Design review of the part built by this model. Coordinates are the model's own, in mm. A direction names the side the tool comes from. Coordinates: 2 decimals unless noted, no trailing zeros. Order: outer loops, then holes, each group sorted by start corner. A loop starts at its lowest first (then second) coordinate and runs counter-clockwise, first axis right, second up. Notation, with made-up numbers: (37, 38.5) -> (90, 38.5) arc R23 cw to (90, 69.5) -> close; hole circle Ø5 at (27.5, -24.75). An arc over 180 degrees is marked (long way). Write item = value, one per line.
Autodesk Inventor part; units mm, degrees
ref_plane "YZ Plane" through (0, 0, 0) normal (1, 0, 0) x (0, 1, 0)
ref_plane "XZ Plane" through (0, 0, 0) normal (0, 1, 0) x (-1, 0, 0)
ref_plane "XY Plane" through (0, 0, 0) normal (0, 0, 1) x (1, 0, 0)
sketch "Sketch1" plane through (0, 0, 0) normal (1, 0, 0) x (0, 1, 0)
  line L0 (38, 32.5) -> (0, 32.5)
  line L1 (0, 32.5) -> (0, -32.5)
  line L2 (0, -32.5) -> (38, -32.5)
  line L3 (0, 0) -> (16.8405, 0)
  line L4 (38, 32.5) -> (38, 27.5)
  line L5 (29, 27.5) -> (5, 27.5)
  line L6 (5, 27.5) -> (5, -27.5)
  line L7 (5, -27.5) -> (29, -27.5)
  line L8 (5.264, 15) -> (-3.604, 15) construction
  line L9 (5.264, -15) -> (-3.604, -15) construction
  line L10 (38, 27.5) -> (36.5301, 27.5)
  line L11 (29, 30) -> (29, 27.5)
  line L12 (36.5301, 27.5) -> (32.2, 30)
  line L13 (32.2, 30) -> (29, 30)
  line L14 (38, -32.5) -> (38, -27.5)
  line L15 (38, -27.5) -> (36.5301, -27.5)
  line L16 (29, -30) -> (29, -27.5)
  line L17 (36.5301, -27.5) -> (32.2, -30)
  line L18 (32.2, -30) -> (29, -30)
  dimension "d0" = 5
  dimension "d1" = 30
  dimension "d2" = 65
  dimension "d3" = 38
  dimension "d5" = 3.2
  dimension "d6" = 24
  dimension "d7" = 2.5
  dimension "d8" = 30
  dimension "d9" = 5
  dimension "d10" = 5
  dimension "d30" = 60
extrude "Extrusion1" add sketch "Sketch1" along normal mid plane 15.1
sketch "Sketch2" plane through (7.55, 0, 0) normal (1, 0, 0) x (0, 0, -1)
  line L0 (32.5, 38) -> (27.5, 38)
  line L1 (27.5, 38) -> (27.5, 36.5301)
  line L2 (27.5, 36.5301) -> (30, 32.2)
  line L3 (30, 32.2) -> (30, 29)
  line L4 (30, 29) -> (27.5, 29)
  line L5 (27.5, 29) -> (27.5, 5)
  line L6 (27.5, 5) -> (-27.5, 5)
  line L7 (-27.5, 5) -> (-27.5, 29)
  line L8 (-27.5, 29) -> (-30, 29)
  line L9 (-30, 29) -> (-30, 32.2)
  line L10 (-30, 32.2) -> (-27.5, 36.5301)
  line L11 (-27.5, 36.5301) -> (-27.5, 38)
  line L12 (-27.5, 38) -> (-32.5, 38)
  line L13 (-32.5, 38) -> (-32.5, 0)
  line L14 (-32.5, 0) -> (32.5, 0)
  line L15 (32.5, 0) -> (32.5, 38)
  line L16 (-30, 32.2) -> (-27.5, 36.5301)
  line L17 (-27.5, 5) -> (-27.5, 29)
  line L18 (-27.5, 36.5301) -> (-27.5, 29)
  line L19 (27.5, 38) -> (27.5, 36.5301)
  line L20 (27.5, 29) -> (27.5, 5)
  line L21 (27.5, 36.5301) -> (27.5, 29)
  point P0 (0, 0)
extrude "Extrusion2" add sketch "Sketch2" along normal blind 2
mirror "Mirror1" about plane through (0, 0, 0) normal (1, 0, 0) of "Extrusion2"
fillet "Fillet1" radius 6 2 edges at (0, 5, 27.5) (0, 5, -27.5)
sketch "Sketch3" plane through (9.55, 0, -32.5) normal (0, -1, 0) x (1, 0, 0)
  line L0 (-9.55, 32.5) -> (28.6439, 32.5)
  point P0 (-9.55, 47.5)
  point P1 (-9.55, 17.5)
  dimension "d16" = 30
hole "Hole1" at (0, 0, 15) at (0, 0, -15) direction (0, 1, 0) diameter 5.5 end through all
fillet "Fillet2" radius 2 2 edges at (0, 38, 27.5) (0, 38, -27.5)
sketch "Sketch4" plane through (-9.55, 5, -21.5) normal (0, 1, 0) x (1, 0, 0)
  line L0 (15.05, -13) -> (4.05, -13)
  line L1 (4.05, -13) -> (4.05, -30)
  line L2 (4.05, -30) -> (15.05, -30)
  line L3 (15.05, -30) -> (15.05, -13)
  point P0 (9.55, -21.5)
  point P1 (15.05, -21.5)
  point P2 (9.55, -13)
  dimension "d25" = 17
  dimension "d26" = 11
extrude "Extrusion3" cut sketch "Sketch4" against normal through all
fillet "Fillet3" radius 2 4 edges at (5.5, 2.5, -8.5) (-5.5, 2.5, -8.5) (-5.5, 2.5, 8.5) (5.5, 2.5, 8.5)
properties part number "Base_Lower_v3"
(1) We need section C-C (x = 0). Give the number of separate pieces and of enclosed holes in the cut face, and give its area (3 significant figures).
Report:
separate_pieces = 4
enclosed_holes = 0
area = 502 mm²
(2) For L1, parallel to Z at x = 0, y = 2.1; L2, parallel to Z at x = 4.5, y = 19; L3, parallel to X at y = 3, z = -15, list the stretches that pass through material, from the lowest coordinate up.
Report:
L1 = -32.5 to -17.75, -12.25 to -8.5, 8.5 to 12.25, 17.75 to 32.5
L2 = -32.5 to -27.5, 27.5 to 32.5
L3 = -9.55 to -2.75, 2.75 to 9.55
(3) We need section B-B (y = 30). Write out the cut boundary in (x, z), and give its area (4 significant figures).
Report:
outline = (-9.55, -32.5) -> (9.55, -32.5) -> (9.55, -27.5) -> (7.55, -27.5) -> (7.55, -30) -> (-7.55, -30) -> (-7.55, -27.5) -> (-9.55, -27.5) -> close; (-9.55, 27.5) -> (-7.55, 27.5) -> (-7.55, 30) -> (7.55, 30) -> (7.55, 27.5) -> (9.55, 27.5) -> (9.55, 32.5) -> (-9.55, 32.5) -> close
area = 115.5 mm²
(4) For faces 1 (the flat face through (0, 31, -30)), 2 (the flat face through (-7, 5, 0)), 3 (the flat face through (0, 38, -31)), 4 (the cylindrical face through (-4.9, 2.46, 7.93)), 5 (the flat face through (-9.55, 4, -3)), list the 3-axis set-ups (+Z, -Z, +X, -X, +Y, -Y) from which the entire face can be reached by the end or side of a thin tool; tool diameter is ignored.
Report:
face_1 = none
face_2 = +X, -X, +Y
face_3 = +Z, -Z, +X, -X, +Y
face_4 = +Y, -Y
face_5 = +Z, -Z, -X, +Y, -Y
(5) Insertion check: pin 1 (6 mm diameter, centred on x = 6, z = 9, fed in from +Y); pin 2 (2 mm diameter, centred on x = -1.5, z = 26, fed in from +Y); pin 3 (0.8 mm diameter, centred on x = 1, z = -28.5, fed in from +Y). Each pin has a flat end and moves straight along its axis. Give the tip position at first contact, or say it passes through.
Report:
pin_1 = 5
pin_2 = 8.6
pin_3 = 37.91
(6) The part is to be moulded in two halves that separate along Y. For faces 6 (the flat face through (0, 31, 30)), 7 (the flat face through (-7, 0, 0)), 8 (the cylindrical face through (0.134, 6.711, -25.696)), say which applies: released by +Y, released by -Y, zero draft, split by the parting line, or undercut.
Report:
face_6 = undercut
face_7 = released by -Y
face_8 = released by +Y
(7) We need section A-A (z = -2.5). Write out the cut boundary in (x, y).
Report:
outline = (-9.55, 0) -> (-5.5, 0) -> (-5.5, 5) -> (-9.55, 5) -> close; (5.5, 0) -> (9.55, 0) -> (9.55, 5) -> (5.5, 5) -> close
(8) We need section D-D (z = -15). Write out the cut boundary in (x, y).
Report:
outline = (-9.55, 0) -> (-2.75, 0) -> (-2.75, 5) -> (-9.55, 5) -> close; (2.75, 0) -> (9.55, 0) -> (9.55, 5) -> (2.75, 5) -> close
